Can you work these out from the model? Positions are in its coordinate system, mm. Face numbers are marked on the shaded views. A direction names the side the tool comes from. Give positions to 0.01 mm unless a question says otherwise; leave off trailing zeros. Loops run counter-clockwise (first coordinate to the right, second up) from the corner with the lowest first, then second, coordinate; pieces in that order, holes last.
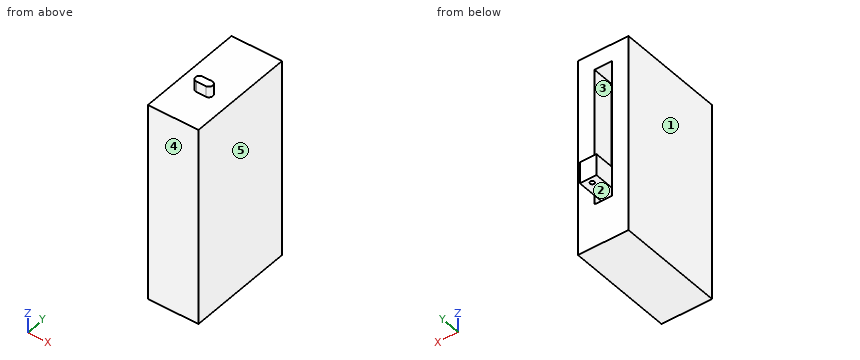
from build123d import *

# Parameters (mm, degrees)
SKETCH1_W           = 7.366
SKETCH1_H           = 29.0322
BOSS_EXTRUDE1_DEPTH = 15.748
SKETCH2_W           = 2.54
SKETCH2_H           = 20.1422
CUT_EXTRUDE1_DEPTH  = 3.175
SKETCH3_W           = 2.4257
SKETCH3_H           = 3.1369
BOSS_EXTRUDE2_DEPTH = 6.0198
SKETCH4_R           = 0.3175
CUT_EXTRUDE2_DEPTH  = 29.596136272
BOSS_EXTRUDE3_DEPTH = 1.5875


with BuildPart() as part:
    # Sketch1 → Boss-Extrude1 (new body)
    with BuildSketch(Plane(origin=(0, 0, 0), x_dir=(1, 0, 0), z_dir=(0, 1, 0))):
        Rectangle(SKETCH1_W, SKETCH1_H)
    extrude(amount=BOSS_EXTRUDE1_DEPTH)

    # Sketch2 → Cut-Extrude1 (cut)
    with BuildSketch(Plane(origin=(0, 15.748, 0), x_dir=(1, 0, 0), z_dir=(0, 1, 0))):
        with Locations((0, -1.905)):
            Rectangle(SKETCH2_W, SKETCH2_H)
    extrude(amount=-CUT_EXTRUDE1_DEPTH, mode=Mode.SUBTRACT)

    # Sketch3 → Boss-Extrude2 (add)
    with BuildSketch(Plane(origin=(0, 12.573, 0), x_dir=(1, 0, 0), z_dir=(0, 1, 0))):
        with Locations((0, 5.32765)):
            Rectangle(SKETCH3_W, SKETCH3_H)
    extrude(amount=BOSS_EXTRUDE2_DEPTH)

    # Sketch4 → Cut-Extrude2 (cut, through all)
    with BuildSketch(Plane(origin=(0, 0, -6.8961), x_dir=(-1, 0, 0), z_dir=(0, 0, -1))):
        with Locations((0, 17.79905)):
            Circle(SKETCH4_R)
    extrude(amount=-CUT_EXTRUDE2_DEPTH, mode=Mode.SUBTRACT)

    # Sketch5 → Boss-Extrude3 (add)
    with BuildSketch(Plane.XY.offset(14.5161)):
        with BuildLine():
            Line((-0.682666257, 6.414003725), (0.682666257, 6.414003725))
            ThreePointArc((0.682666257, 6.414003725), (1.254669982, 5.842), (0.682666257, 5.269996275))
            Line((0.682666257, 5.269996275), (-0.682666257, 5.269996275))
            ThreePointArc((-0.682666257, 5.269996275), (-1.254669982, 5.842), (-0.682666257, 6.414003725))
        make_face()
    extrude(amount=BOSS_EXTRUDE3_DEPTH)


solid = part.part
(1) Please list where these lines run through material, in increasing order: probe 1 along Z at (x, y) = (1, 15.25); probe 2 along Y at (x, z) = (0, -6); probe 3 along Y at (x, z) = (0.25, -11.5).
Returned:
probe 1: z = -14.52 to -8.17, -6.9 to -3.76, 11.98 to 14.52
probe 2: y = 0 to 17.48, 18.12 to 18.59
probe 3: y = 0 to 15.75
(2) Will these pins go through, and if not, where does the flat tip stop? P1, Ø0.8, axis at x = -0.5, y = 14.5, coming from the +Z side; P2, Ø1.5, axis at x = -2.5, z = -6, coming from the -Y side; P3, Ø4, axis at x = 2, z = 8, coming from the +Y side; P4, Ø0.7, axis at x = 0, y = 16.5, coming from the +Z side.
Returned:
P1: stops at z = 14.52
P2: stops at y = 0
P3: stops at y = 15.75
P4: stops at z = -3.76
(3) Suppose I cut it at D-D on x = -2. List the corners of the cut face in (y, z) for me, plus the area to 3 significant figures.
Returned:
outline: (0, -14.52) - (15.75, -14.52) - (15.75, 14.52) - (0, 14.52) - close
area: 457 mm2
(4) Thinking about a two-plate mould opening in X: for the marked faces 3, 4 and 5, which applies, pulls with the +X half, pulls with the -X half, needs draft (parallel to the pull), parting line crosses it, or undercut?
Returned:
face 3: undercut
face 4: needs draft
face 5: pulls with the +X half
(5) Suppose I cut it at B-B on x = 0. List the corners of the cut face in (y, z) for me, plus the area to 3 significant figures.
Returned:
outline: (0, -14.52) - (15.75, -14.52) - (15.75, -8.17) - (12.57, -8.17) - (12.57, -6.9) - (17.48, -6.9) - (17.48, -3.76) - (12.57, -3.76) - (12.57, 11.98) - (15.75, 11.98) - (15.75, 14.52) - (6.41, 14.52) - (6.41, 16.1) - (5.27, 16.1) - (5.27, 14.52) - (0, 14.52) - close; (18.12, -6.9) - (18.59, -6.9) - (18.59, -3.76) - (18.12, -3.76) - close
area: 412 mm2
(6) Suppose I cut it at A-A on y = 14.25. List the corners of the cut face in (x, z) for me, plus the area to 3 significant figures.
Returned:
outline: (-3.68, -14.52) - (3.68, -14.52) - (3.68, 14.52) - (-3.68, 14.52) - close; (-1.21, -6.9) - (1.21, -6.9) - (1.21, -3.76) - (-1.21, -3.76) - close; hole (-1.27, -8.17) - (1.27, -8.17) - (1.27, 11.98) - (-1.27, 11.98) - close
area: 170 mm2
(7) Suppose I cut it at C-C on z = 4.5. List the corners of the cut face in (x, y) for me.
Returned:
outline: (-3.68, 0) - (3.68, 0) - (3.68, 15.75) - (1.27, 15.75) - (1.27, 12.57) - (-1.27, 12.57) - (-1.27, 15.75) - (-3.68, 15.75) - close
(8) Which directions (+Z, -Z, +X, -X, +Y, -Y) give clear straight access to the entire face, cutting with the end or side of a thin tool? Please do the marked faces 1 and 2.
Returned:
face 1: +Z, -Z, -X, +Y, -Y
face 2: +Y
